Build history of the part. All positions in model axes, mm. Face numbers are marked on the shaded views. Round coordinates to 2 decimals unless told otherwise and drop trailing zeros. Loops run counter-clockwise (first coordinate to the right, second up) from the corner with the lowest first, then second, coordinate; pieces in that order, holes last. Notation, with made-up numbers: (-1, -18) - (28, -18) arc R18 ccw to (28, 15) - close; hole circle Ø4 at (-37, 79). An arc over 180 degrees is marked (long way). Use a Markdown table: item, result.
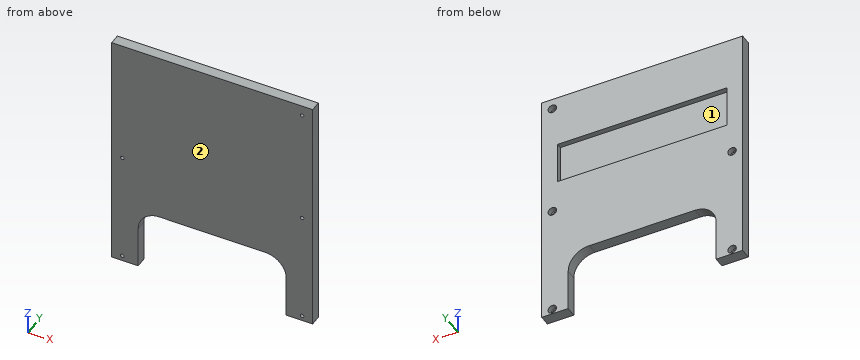
from build123d import *

# Parameters (mm, degrees)
SKETCH1_W                       = 120.65
SKETCH1_H                       = 146.05
BOSS_EXTRUDE1_DEPTH             = 6.35
SKETCH7_R                       = 2.54
CUT_EXTRUDE1_DEPTH              = 3.175
F_2_CLEARANCE_HOLE2_D           = 2.159
F_2_CLEARANCE_HOLE2_CSINK_D     = 3.429
F_2_CLEARANCE_HOLE2_CSINK_ANGLE = 75
SKETCH13_W                      = 88.9
SKETCH13_H                      = 38.1
CUT_EXTRUDE3_DEPTH              = 95.931969062
FILLET1_R                       = 12.7
SKETCH11_W                      = 101.6
SKETCH11_H                      = 25.4
CUT_EXTRUDE2_DEPTH              = 3.175


with BuildPart() as part:
    # Sketch1 → Boss-Extrude1 (new body)
    with BuildSketch(Plane(origin=(0, 0, 0), x_dir=(1, 0, 0), z_dir=(0, 1, 0))):
        Rectangle(SKETCH1_W, SKETCH1_H)
    extrude(amount=BOSS_EXTRUDE1_DEPTH)

    # Sketch7 → Cut-Extrude1 (cut)
    with BuildSketch(Plane(origin=(0, 6.35, 0), x_dir=(1, 0, 0), z_dir=(0, 1, 0))):
        with Locations(Location((-53.975, 3.175, 0), (0, 0, 270))):
            Circle(SKETCH7_R)
        with Locations(Location((53.975, 3.175, 0), (0, 0, 270))):
            Circle(SKETCH7_R)
        with Locations(Location((53.975, -66.675, 0), (0, 0, 270))):
            Circle(SKETCH7_R)
        with Locations(Location((-53.975, 69.85, 0), (0, 0, 270))):
            Circle(SKETCH7_R)
        with Locations(Location((53.975, 69.85, 0), (0, 0, 270))):
            Circle(SKETCH7_R)
    extrude(amount=-CUT_EXTRUDE1_DEPTH, mode=Mode.SUBTRACT)

    # #2 Clearance Hole2 (through all)
    with Locations(Plane(origin=(0, 3.175, 0), x_dir=(1, 0, 0), z_dir=(0, 1, 0))):
        with Locations((-53.975, 3.175), (53.975, 3.175), (53.975, -66.675), (-53.975, 69.85), (53.975, 69.85)):
            CounterSinkHole(F_2_CLEARANCE_HOLE2_D / 2, F_2_CLEARANCE_HOLE2_CSINK_D / 2, counter_sink_angle=F_2_CLEARANCE_HOLE2_CSINK_ANGLE)

    # Sketch13 → Cut-Extrude3 (cut, through all)
    with BuildSketch(Plane(origin=(0, 6.35, 0), x_dir=(1, 0, 0), z_dir=(0, 1, 0))):
        with Locations((0, 53.975)):
            Rectangle(SKETCH13_W, SKETCH13_H)
    extrude(amount=-CUT_EXTRUDE3_DEPTH, mode=Mode.SUBTRACT)

    # Fillet1
    fillet1_edges = [part.edges().sort_by_distance(p)[0] for p in [
        (44.45, 3.175, -34.925),
        (-44.45, 3.175, -34.925),
    ]]
    fillet(fillet1_edges, radius=FILLET1_R)

    # Sketch11 → Cut-Extrude2 (cut)
    with BuildSketch(Plane(origin=(0, 6.35, 0), x_dir=(1, 0, 0), z_dir=(0, 1, 0))):
        with Locations((0, -28.575)):
            Rectangle(SKETCH11_W, SKETCH11_H)
    extrude(amount=-CUT_EXTRUDE2_DEPTH, mode=Mode.SUBTRACT)


solid = part.part
Q1. Cut at B-B, the plane x = 14.5. List the corners of the cut face in (y, z) (3 decimals).
Results found:
| item | result |
|---|---|
| outline | (0, -34.925) - (6.35, -34.925) - (6.35, 15.875) - (3.175, 15.875) - (3.175, 41.275) - (6.35, 41.275) - (6.35, 73.025) - (0, 73.025) - close |
Q2. Cut at A-A, the plane z = -56. List the corners of the cut face in (x, y) (3 decimals), plus the area to 3 significant figures.
Results found:
| item | result |
|---|---|
| outline | (-60.325, 0) - (-44.45, 0) - (-44.45, 6.35) - (-60.325, 6.35) - close; (44.45, 0) - (60.325, 0) - (60.325, 6.35) - (44.45, 6.35) - close |
| area | 202 mm2 |
Q3. Cut at C-C, the plane x = 48.5. List the corners of the cut face in (y, z) (3 decimals).
Results found:
| item | result |
|---|---|
| outline | (0, -73.025) - (6.35, -73.025) - (6.35, 15.875) - (3.175, 15.875) - (3.175, 41.275) - (6.35, 41.275) - (6.35, 73.025) - (0, 73.025) - close |
Q4. Pull direction X, two halves, no side cores. Call the marked faces 1 and 2: pulls with the +X half, pulls with the -X half, needs draft (parallel to the pull), parting line crosses it, or undercut.
Results found:
| item | result |
|---|---|
| face 1 | undercut |
| face 2 | needs draft |
Q5. Drop flat-ended pins along their axis: pin 1 (2.5 mm diameter, centred on x = 53.975, z = -3.175, fed in from +Y); pin 2 (2.5 mm diameter, centred on x = 20, y = 5, fed in from -Z) (3 decimals); pin 3 (1.7 mm diameter, centred on x = 53.975, z = -69.85, fed in from -Y). Give the stop position or say it passes through.
Results found:
| item | result |
|---|---|
| pin 1 | stops at y = 2.57 |
| pin 2 | stops at z = -34.925 |
| pin 3 | passes through |
Q6. Probe line 1 (X direction, y = 4.55, z = -69.85) (3 decimals); line 2 (Z direction, x = -21, y = 5.75) (3 decimals); line 3 (Z direction, x = -52, y = 4) (3 decimals). List the from-to ranges inside material, lowest first.
Results found:
| item | result |
|---|---|
| line 1 | x = -60.325 to -56.515, -51.435 to -44.45, 44.45 to 51.435, 56.515 to 60.325 |
| line 2 | z = -34.925 to 15.875, 41.275 to 73.025 |
| line 3 | z = -73.025 to -71.447, -68.253 to -4.772, -1.578 to 73.025 |
